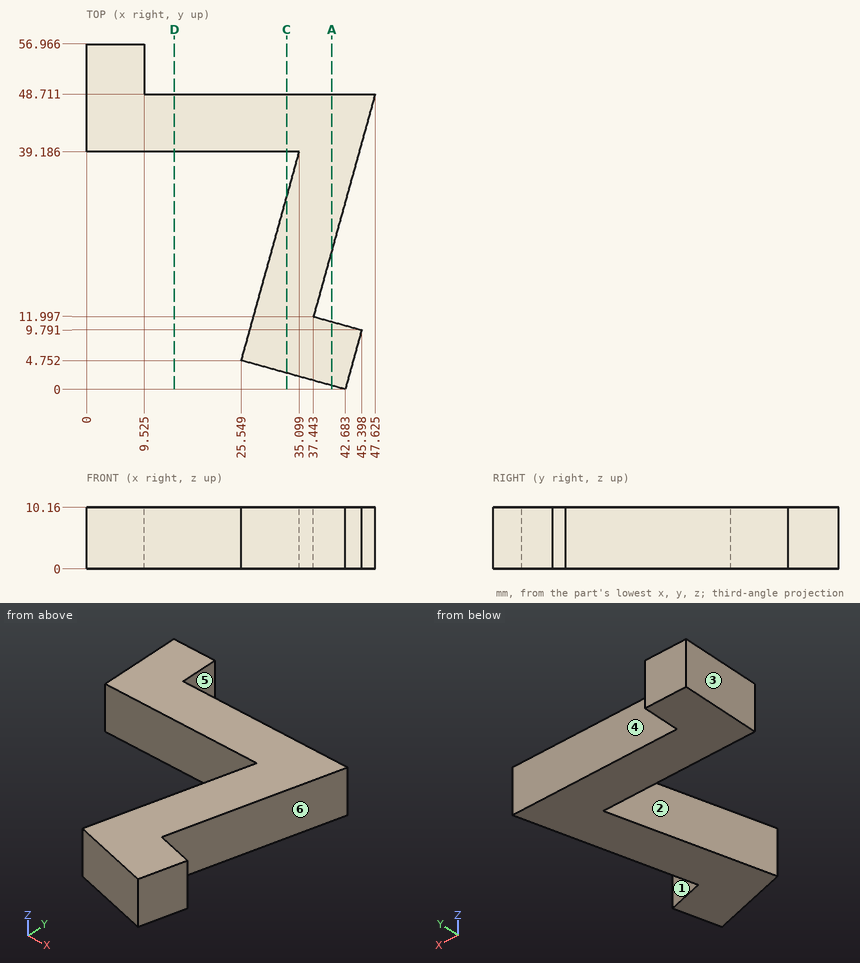
Design review of the part shown in the three views and the two pictorial views. Dimensions are in mm from the part's minimum x, y and z. A direction names the side the tool comes from. Coordinates: 2 decimals unless noted, no trailing zeros. Order: outer loops, then holes, each group sorted by start corner. A loop starts at its lowest first (then second) coordinate and runs counter-clockwise, first axis right, second up. Notation, with made-up numbers: (34.5, -9) - (79.5, -9) arc R21 cw to (79.5, 13) - close; hole circle Ø6 at (-19, -8.5). An arc over 180 degrees is marked (long way). One line per question, with ' | ' between items.
Q1. Consider section D-D, the plane x = 14.5. Give the boundary of the cut face in (y, z) (1 decimal).
Answer key:
outline: (39.2, 0) - (48.7, 0) - (48.7, 10.2) - (39.2, 10.2) - close
Q2. Clearance check with flat-ended pins moving along their axes: pin 1 Ø12 at (x, y) = (12.5, 46.5) entering from -Z; pin 2 Ø3 at (x, z) = (36.5, 5.5) entering from +Y; pin 3 Ø3 at (y, z) = (21, 1.5) entering from +X; pin 4 Ø5 at (x, z) = (14.5, 6.5) entering from -Y. State where each tip first meets the part, or that it passes through.
Answer key:
pin 1: stops at z = 0 | pin 2: stops at y = 48.71 | pin 3: stops at x = 40.36 | pin 4: stops at y = 39.19
Q3. For the marked faces 1, 2 and 3, list the 3-axis set-ups (+Z, -Z, +X, -X, +Y, -Y) from which the entire face can be reached by the end or side of a thin tool; tool diameter is ignored.
Answer key:
face 1: +Z, -Z, +X | face 2: +Z, -Z, -X | face 3: +Z, -Z, -X, +Y, -Y
Q4. The part is to be moulded in two halves that separate along Y. For the marked faces 4, 5 and 6, say which applies: +Y half, -Y half, draft (parallel to the pull), parting line (faces both ways), or undercut.
Answer key:
face 4: +Y half | face 5: draft | face 6: undercut
Q5. To check wall thickness, follow line 1 along Y through (x, z) = (13, 8) (1 decimal); line 2 along Y through (x, z) = (2, 9.5) (1 decimal); line 3 along X through (y, z) = (52, 6) (1 decimal). State the ranges of each line that lie inside material, in increasing order.
Answer key:
line 1: y = 39.2 to 48.7 | line 2: y = 39.2 to 57 | line 3: x = 0 to 9.5
Q6. Consider section C-C, the plane x = 33. Give the boundary of the cut face in (y, z) (1 decimal), then the cut area to 3 significant figures.
Answer key:
outline: (2.7, 0) - (31.6, 0) - (31.6, 10.2) - (2.7, 10.2) - close; (39.2, 0) - (48.7, 0) - (48.7, 10.2) - (39.2, 10.2) - close | area: 391 mm2
Q7. Consider section A-A, the plane x = 40.5. Give the boundary of the cut face in (y, z) (1 decimal), then the cut area to 3 significant figures.
Answer key:
outline: (0.6, 0) - (11.1, 0) - (11.1, 10.2) - (0.6, 10.2) - close; (23, 0) - (48.7, 0) - (48.7, 10.2) - (23, 10.2) - close | area: 368 mm2
